from build123d import *

# Parameters (mm, degrees)
F1_DEPTH = 2


with BuildPart() as f1:
    # F0 (on Front) → F1 (new body)
    with BuildSketch(Plane.XZ):
        Polygon((-39.375, 0), (0, 0), (39.375, 0), (44.658148, 70), (32.658148, 70), (29.261839, 25), (-29.506019, 25), (-33.341852, 70), (-45.341852, 70), align=None)
        Polygon((18.75, 9), (0, 9), (-18.75, 9), (-18.75, 11), (18.75, 11), align=None, mode=Mode.SUBTRACT)
    extrude(amount=F1_DEPTH)


solid = f1.part
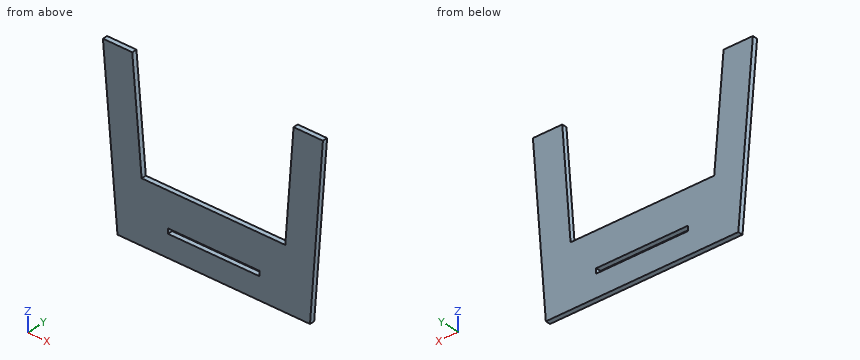
Could you check a few things on this model? Use its own coordinates, in mm. Give positions to 0.01 mm unless a question says otherwise; leave off trailing zeros. Loops run counter-clockwise (first coordinate to the right, second up) from the corner with the lowest first, then second, coordinate; pieces in that order, holes last. Notation, with made-up numbers: M 84.25,-22 L 111.25,-22 A18 ccw 111.25,2 Z; hole C 1.25,74.25 d8. An arc over 180 degrees is marked long. Answer as a JSON object with one key per item and string values.
Q1. For P1, Ø1, axis at y = -1, z = 10, coming from the -X side; P2, Ø1, axis at x = 2, y = -1.5, coming from the +Z side, each with a flat end and sliding along its axis, tell me the tip position at first contact or that it passes through.
Values found:
{"P1": "stops at x = -40.27", "P2": "stops at z = 25"}
Q2. Suppose I cut it at A-A, the plane x = -13. List the corners of the cut face in (y, z) for me, plus the area to 3 significant figures.
Values found:
{"outline": "M -2,0 L 0,0 L 0,9 L -2,9 Z; M -2,11 L 0,11 L 0,25 L -2,25 Z", "area": "46.0 mm²"}
Q3. Suppose I cut it at D-D, the plane x = -23. List the corners of the cut face in (y, z) for me.
Values found:
{"outline": "M -2,0 L 0,0 L 0,25 L -2,25 Z"}
Q4. Suppose I cut it at C-C, the plane y = -1.5. List the corners of the cut face in (x, z) for me (3 decimals).
Values found:
{"outline": "M -45.342,70 L -39.375,0 L 39.375,0 L 44.658,70 L 32.658,70 L 29.262,25 L -29.506,25 L -33.342,70 Z; hole M -18.75,9 L 18.75,9 L 18.75,11 L -18.75,11 Z"}
Q5. Suppose I cut it at B-B, the plane z = 54. List the corners of the cut face in (x, y) for me, plus the area to 3 significant figures.
Values found:
{"outline": "M -43.98,-2 L -31.98,-2 L -31.98,0 L -43.98,0 Z; M 31.45,-2 L 43.45,-2 L 43.45,0 L 31.45,0 Z", "area": "48.0 mm²"}
Q6. If I drill on probe 1 along Z at (x, y) = (6, -0.4); probe 2 along Z at (x, y) = (-22, -0.5); probe 3 along X at (y, z) = (-0.85, 43), over which ranges is the centre line in solid material (lowest first)? Write a range as [from, to].
Values found:
{"probe 1": "z = [0, 9], [11, 25]", "probe 2": "z = [0, 25]", "probe 3": "x = [-43.04, -31.04], [30.62, 42.62]"}
